from build123d import *

# Parameters (mm, degrees)
SKETCH1_W           = 398.88
SKETCH1_H           = 100
BOSS_EXTRUDE1_DEPTH = 500
BOSS_EXTRUDE2_DEPTH = 698.88


with BuildPart() as part:
    # Sketch1 → Boss-Extrude1 (new body)
    with BuildSketch(Plane.XY):
        with Locations((-24.459622642, 226.581886792)):
            Rectangle(SKETCH1_W, SKETCH1_H)
    extrude(amount=BOSS_EXTRUDE1_DEPTH)

    # Sketch2 → Boss-Extrude2 (add)
    with BuildSketch(Plane.ZY.offset(373.899622642)):
        with BuildLine():
            Line((500, 276.581886792), (500, 176.581886792))
            Line((500, 176.581886792), (485, 176.581886792))
            Line((485, 176.581886792), (485, 152.581886792))
            ThreePointArc((485, 152.581886792), (530.001319942, 126.601886792), (485, 100.621886792))
            Line((485, 100.621886792), (485, 77.731886792))
            ThreePointArc((485, 77.731886792), (599.838299174, 169.059957008), (500, 276.581886792))
        make_face()
    extrude(amount=-BOSS_EXTRUDE2_DEPTH)


solid = part.part
Model file for the job. Use its own axes, mm. A direction names the side the tool comes from. Coordinates: 2 decimals unless noted, no trailing zeros. Order: outer loops, then holes, each group sorted by start corner. A loop starts at its lowest first (then second) coordinate and runs counter-clockwise, first axis right, second up. Notation, with made-up numbers: (53.25, -4.75) -> (96.25, -4.75) arc R28 cw to (96.25, 17.25) -> close; hole circle Ø10 at (36.25, 56). An arc over 180 degrees is marked (long way). Return JSON: item names as keys, results as strings. Group by question number.
Item 1: Saw through at D-D on x = 214. Write the cut outline in (y, z), then the cut area to 3 significant figures.
Item 2: Wall check: line 1 along X through (y, z) = (245, 217); line 2 along Y through (x, z) = (-54.5, 304); line 3 along Y through (x, z) = (-296, 519). Give the ranges that are in metal, low to high. Write a range as [from, to].
Item 3: Saw through at A-A on x = 116. Write the cut outline in (y, z), then the cut area to 3 significant figures.
Item 4: Saw through at C-C on z = 360.5. Write the cut outline in (x, y).
Item 5: Pull direction Z, two halves, no side cores. Call faces 1 (the cylindrical face through (-29, 127, 530)), 2 (the flat face through (-29, 89, 485)), 3 (the flat face through (324.98, 178, 542)): pulls with the +Z half, pulls with the -Z half, needs draft (parallel to the pull), parting line crosses it, or undercut.
Item 6: Flat gauge pins, fed straight in: P1, Ø25, axis at x = 10, y = 94.5, coming from the -Z side; P2, Ø2, axis at x = 152.5, z = 258.5, coming from the -Y side; P3, Ø4.5, axis at x = -296.5, z = 496, coming from the +Y side. Where does each tip first touch, or does it go through?
Item 7: Saw through at B-B on y = 252.5. Write the cut outline in (x, z), then the cut area to 3 significant figures.
Item 8: Tool access for faces 4 (the flat face through (249, 176.582, 493)), 5 (the flat face through (-300, 176.582, 493)), 6 (the flat face through (-27, 176.582, 239)): list every direction of +Z, -Z, +X, -X, +Y, -Y with a clear straight run to the whole face (end or side of a thin tool).
Values found:
{
 "1": {"outline": "(77.73, 485) -> (100.62, 485) arc R30 cw (long way) to (152.58, 485) -> (176.58, 485) -> (176.58, 500) -> (276.58, 500) arc R100 ccw (long way) to start", "area": "15,000 mm2"},
 "2": {"line 1": "x = [-223.9, 174.98]", "line 2": "y = [176.58, 276.58]", "line 3": "y = [78.38, 103.38], [149.82, 274.78]"},
 "3": {"outline": "(77.73, 485) -> (100.62, 485) arc R30 cw (long way) to (152.58, 485) -> (176.58, 485) -> (176.58, 0) -> (276.58, 0) -> (276.58, 500) arc R100 ccw (long way) to start", "area": "65,000 mm2"},
 "4": {"outline": "(-223.9, 176.58) -> (174.98, 176.58) -> (174.98, 276.58) -> (-223.9, 276.58) -> close"},
 "5": {"face 1": "undercut", "face 2": "pulls with the -Z half", "face 3": "needs draft"},
 "6": {"P1": "stops at z = 485", "P2": "stops at y = 176.58", "P3": "stops at y = 176.58"},
 "7": {"outline": "(-373.9, 500) -> (-223.9, 500) -> (-223.9, 0) -> (174.98, 0) -> (174.98, 500) -> (324.98, 500) -> (324.98, 565.21) -> (-373.9, 565.21) -> close", "area": "245,000 mm2"},
 "8": {"face 4": "-Z, +X, +Y", "face 5": "-Z, -X, +Y", "face 6": "-Z, +X, -X, -Y"}
}
